Work out the finished part from the listing and answer in its coordinate system (mm). A direction names the side the tool comes from. Give positions to 0.01 mm unless a question says otherwise; leave off trailing zeros. Order: outer loops, then holes, each group sorted by start corner. A loop starts at its lowest first (then second) coordinate and runs counter-clockwise, first axis right, second up. Notation, with made-up numbers: (-4.75, 26.5) -> (0.25, 26.5) arc R20 cw to (0.25, 52.5) -> close; hole circle Ø9 at (-14, 32.5). An arc over 180 degrees is marked (long way). Use a Markdown table: item, result. Add a question column.
```python
from build123d import *

# Parameters (mm, degrees)
BOSS_EXTRU_1_DEPTH             = 1.99
ESQUISSE3_W                    = 5.82
ESQUISSE3_H                    = 9.63
BOSS_EXTRU_5_DEPTH             = 6.93
R_P_TITION_LIN_AIRE2_COUNT     = 3
R_P_TITION_LIN_AIRE2_PITCH     = 18.509
R_P_TITION_LIN_AIRE2_COL_COUNT = 3
R_P_TITION_LIN_AIRE2_COL_PITCH = 18.509
D_GAGEMENT_M31_D               = 3.6


with BuildPart() as part:
    # Esquisse2 → Boss.-Extru.1 (new body)
    with BuildSketch(Plane.XY):
        with BuildLine():
            Line((-46.628094051, 77.059557029), (71.371905949, 77.059557029))
            ThreePointArc((71.371905949, 77.059557029), (73.493226293, 76.180877372), (74.371905949, 74.059557029))
            Line((74.371905949, 74.059557029), (74.371905949, 50.059557029))
            ThreePointArc((74.371905949, 50.059557029), (73.493226293, 47.938236685), (71.371905949, 47.059557029))
            Line((71.371905949, 47.059557029), (-46.628094051, 47.059557029))
            ThreePointArc((-46.628094051, 47.059557029), (-48.749414394, 47.938236685), (-49.628094051, 50.059557029))
            Line((-49.628094051, 50.059557029), (-49.628094051, 74.059557029))
            ThreePointArc((-49.628094051, 74.059557029), (-48.749414394, 76.180877372), (-46.628094051, 77.059557029))
        make_face()
    extrude(amount=BOSS_EXTRU_1_DEPTH)

    # Esquisse3 → Boss.-Extru.5 (add)
    with BuildSketch(Plane(origin=(0, 0, 0), x_dir=(-1, 0, 0), z_dir=(0, 0, -1))):
        with Locations((-12.371905949, 70.244557029)):
            Rectangle(ESQUISSE3_W, ESQUISSE3_H)
    boss_extru_5 = extrude(amount=BOSS_EXTRU_5_DEPTH)

    # Répétition linéaire2: Boss.-Extru.5 ×3
    with Locations(*[(-i * R_P_TITION_LIN_AIRE2_PITCH, 0, 0) for i in range(1, R_P_TITION_LIN_AIRE2_COUNT)]):
        add(boss_extru_5)

    # Répétition linéaire2 col: Boss.-Extru.5 ×3
    with Locations(*[(i * R_P_TITION_LIN_AIRE2_COL_PITCH, 0, 0) for i in range(1, R_P_TITION_LIN_AIRE2_COL_COUNT)]):
        add(boss_extru_5)

    # Dégagement M31 (through all)
    with Locations(Plane(origin=(0, 0, 0), x_dir=(-1, 0, 0), z_dir=(0, 0, -1))):
        with Locations((-41.671905949, 53.239557029), (16.928094051, 53.239557029)):
            Hole(D_GAGEMENT_M31_D / 2)


solid = part.part
```
1) The part is cut by section C-C, the plane y = 71. Determine the outline of the cut face in (x, z).
2) Flat-ended cylindrical pins translate along their axes: pin 1 (3.5 mm diameter, centred on y = 71, z = -3.5, fed in from +X); pin 2 (3 mm diameter, centred on x = 11.5, z = -4, fed in from +Y); pin 3 (4.5 mm diameter, centred on x = 32, z = -4, fed in from -Y). Find the tip coordinate at first contact, or state that the pin passes through.
3) The part is cut by section A-A, the plane z = -4.5. Determine the outline of the cut face in (x, y), then the cut area to 3 significant figures.
4) The part is cut by section D-D, the plane y = 62. Determine the outline of the cut face in (x, z), then the cut area to 3 significant figures.
5) Which of the six approach directions +Z, -Z, +X, -X, +Y, -Y give full straight-line access (tool end or side, diameter ignored) to faces 1 (the flat face through (52.3, 70, -3)), 2 (the flat face through (27.971, 70, -3)), 3 (the flat face through (49, 75.06, -3)), 4 (the flat face through (31, 70, -6.93)), 5 (the flat face through (31, 65.43, -3))?
6) Straight lines are drawn through the part: line 1 (X direction, y = 68, z = -2); line 2 (Z direction, x = -42.5, y = 55); line 3 (Y direction, x = 51, z = -1.25). For each, find the intervals that lie inside material, in ascending order.
7) The part is cut by section B-B, the plane x = 50.5. Determine the outline of the cut face in (y, z).
8) Determine the mould class of faces 6 (the flat face through (-21.736, 70, -3)), 7 (the flat face through (-6, 75.06, -3)), 8 (the cylindrical face through (73.47, 76.204, 0.981)), 9 (the cylindrical face through (-17.318, 51.482, 1.009)) for opening direction X: released by +X, released by -X, zero draft, split by the parting line, or undercut.
A:
| question | item | result |
|---|---|---|
| 1 | outline | (-49.63, 0) -> (-27.56, 0) -> (-27.56, -6.93) -> (-21.74, -6.93) -> (-21.74, 0) -> (-9.05, 0) -> (-9.05, -6.93) -> (-3.23, -6.93) -> (-3.23, 0) -> (9.46, 0) -> (9.46, -6.93) -> (15.28, -6.93) -> (15.28, 0) -> (27.97, 0) -> (27.97, -6.93) -> (33.79, -6.93) -> (33.79, 0) -> (46.48, 0) -> (46.48, -6.93) -> (52.3, -6.93) -> (52.3, 0) -> (74.37, 0) -> (74.37, 1.99) -> (-49.63, 1.99) -> close |
| 2 | pin 1 | x = 52.3 |
| 2 | pin 2 | y = 75.06 |
| 2 | pin 3 | y = 65.43 |
| 3 | outline | (-27.56, 65.43) -> (-21.74, 65.43) -> (-21.74, 75.06) -> (-27.56, 75.06) -> close; (-9.05, 65.43) -> (-3.23, 65.43) -> (-3.23, 75.06) -> (-9.05, 75.06) -> close; (9.46, 65.43) -> (15.28, 65.43) -> (15.28, 75.06) -> (9.46, 75.06) -> close; (27.97, 65.43) -> (33.79, 65.43) -> (33.79, 75.06) -> (27.97, 75.06) -> close; (46.48, 65.43) -> (52.3, 65.43) -> (52.3, 75.06) -> (46.48, 75.06) -> close |
| 3 | area | 280 mm^2 |
| 4 | outline | (-49.63, 0) -> (74.37, 0) -> (74.37, 1.99) -> (-49.63, 1.99) -> close |
| 4 | area | 247 mm^2 |
| 5 | face 1 | -Z, +X, +Y, -Y |
| 5 | face 2 | -Z, +Y, -Y |
| 5 | face 3 | -Z, +X, -X, +Y |
| 5 | face 4 | -Z, +X, -X, +Y, -Y |
| 5 | face 5 | -Z, +X, -X, -Y |
| 6 | line 1 | -27.56 to -21.74, -9.05 to -3.23, 9.46 to 15.28, 27.97 to 33.79, 46.48 to 52.3 |
| 6 | line 2 | 0 to 1.99 |
| 6 | line 3 | 65.43 to 75.06 |
| 7 | outline | (47.06, 0) -> (65.43, 0) -> (65.43, -6.93) -> (75.06, -6.93) -> (75.06, 0) -> (77.06, 0) -> (77.06, 1.99) -> (47.06, 1.99) -> close |
| 8 | face 6 | undercut |
| 8 | face 7 | zero draft |
| 8 | face 8 | released by +X |
| 8 | face 9 | undercut |
